from build123d import *

# Parameters (mm, degrees)
BOSS_EXTRUDE1_DEPTH = 3.175


with BuildPart() as part:
    # Sketch1 → Boss-Extrude1 (new body)
    with BuildSketch(Plane.XY):
        with BuildLine():
            Line((-9.525, 12.7), (9.525, 12.7))
            Line((9.525, 12.7), (9.525, 6.35))
            Line((9.525, 6.35), (12.7, 6.35))
            Line((12.7, 6.35), (12.7, 0.865465632))
            ThreePointArc((12.7, 0.865465632), (9.4234, 0), (12.7, -0.865465632))
            Line((12.7, -0.865465632), (12.7, -6.35))
            Line((12.7, -6.35), (9.525, -6.35))
            Line((9.525, -6.35), (9.525, -12.7))
            Line((9.525, -12.7), (6.35, -12.7))
            Line((6.35, -12.7), (6.35, -9.467093743))
            Line((6.35, -9.467093743), (3.175, -9.467093743))
            Line((3.175, -9.467093743), (3.175, -12.7))
            Line((3.175, -12.7), (0.865465632, -12.7))
            ThreePointArc((0.865465632, -12.7), (0, -9.4234), (-0.865465632, -12.7))
            Line((-0.865465632, -12.7), (-3.175, -12.7))
            Line((-3.175, -12.7), (-3.175, -9.467093743))
            Line((-3.175, -9.467093743), (-6.35, -9.467093743))
            Line((-6.35, -9.467093743), (-6.35, -12.7))
            Line((-6.35, -12.7), (-9.525, -12.7))
            Line((-9.525, -12.7), (-9.525, -6.35))
            Line((-9.525, -6.35), (-12.7, -6.35))
            Line((-12.7, -6.35), (-12.7, -0.865465632))
            ThreePointArc((-12.7, -0.865465632), (-9.4234, 0), (-12.7, 0.865465632))
            Line((-12.7, 0.865465632), (-12.7, 6.35))
            Line((-12.7, 6.35), (-9.525, 6.35))
            Line((-9.525, 6.35), (-9.525, 12.7))
        make_face()
    extrude(amount=BOSS_EXTRUDE1_DEPTH)


solid = part.part
The model under review builds one solid part; all positions refer to its coordinate system, in mm. A direction names the side the tool comes from. Give positions to 0.01 mm unless a question says otherwise; leave off trailing zeros. Write each loop counter-clockwise with the first axis right and the second up, starting at its lowest first coordinate (ties: lowest second). Pieces come first, ordered by that corner, then holes.
1. Tool access review of faces 5 (the flat face through (0, 0, 0)), 6 (the flat face through (2, -12.7, 2)), 7 (the flat face through (-6.35, -11, 2)), 8 (the flat face through (9.525, -9, 2)), 9 (the flat face through (11, 6.35, 2)): name each direction out of +Z, -Z, +X, -X, +Y, -Y from which nothing blocks a thin tool from reaching the whole face with its end or side.
2. Wall thickness on L1, parallel to X at y = -11.25, z = 2.5 (3 decimals); L2, parallel to X at y = 8, z = 0.55 (3 decimals); L3, parallel to Y at x = 3.25, z = 2.5: over which ranges is each line inside the solid? List them lowest first.
3. Draft analysis for pull direction X (two halves, no side actions). For faces 1 (the flat face through (5, -9.467, 2)), 2 (the cylindrical face through (-9.425, -0.064, 1.565)), 3 (the flat face through (-11, 6.35, 2)), 4 (the flat face through (-9.525, 9, 2)), state which applies: +X half, -X half, draft (parallel to the pull), parting line (faces both ways), or undercut.
4. Add section B-B, the plane x = -11. Write out the cut boundary in (y, z) (3 decimals), plus the area to 3 significant figures.
5. Add section C-C, the plane y = 0. Write out the cut boundary in (x, z) (3 decimals), plus the area to 3 significant figures.
6. Add section A-A, the plane z = 1.4. Write out the cut boundary in (x, y) (3 decimals), plus the area to 3 significant figures.
7. Add section D-D, the plane x = 0. Write out the cut boundary in (y, z) (3 decimals), plus the area to 3 significant figures.
8. For P1, Ø1, axis at x = 11, z = 1, coming from the +Y side; P2, Ø1, axis at x = -5, z = 2, coming from the -Y side; P3, Ø5.5, axis at x = 0, y = -11.176, coming from the -Z side; P4, Ø1, axis at y = -11.5, z = 1.5, coming from the +X side (3 decimals), all flat-tipped, find the tip position at first contact; note any pin that passes through.
Worked answers:
1. face 5: -Z, +X, -X, +Y, -Y
1. face 6: +Z, -Z, +X, -X, -Y
1. face 7: +Z, -Z, -Y
1. face 8: +Z, -Z, +X, -Y
1. face 9: +Z, -Z, +X, +Y
2. L1: x = -9.525 to -6.35, -3.175 to -1.751, 1.751 to 3.175, 6.35 to 9.525
2. L2: x = -9.525 to 9.525
2. L3: y = -9.47 to 12.7
3. face 1: undercut
3. face 2: undercut
3. face 3: draft
3. face 4: -X half
4. outline: (-6.35, 0) - (-1.744, 0) - (-1.744, 3.175) - (-6.35, 3.175) - close; (1.744, 0) - (6.35, 0) - (6.35, 3.175) - (1.744, 3.175) - close
4. area: 29.2 mm2
5. outline: (-9.423, 0) - (9.423, 0) - (9.423, 3.175) - (-9.423, 3.175) - close
5. area: 59.8 mm2
6. outline: (-12.7, -6.35) - (-9.525, -6.35) - (-9.525, -12.7) - (-6.35, -12.7) - (-6.35, -9.467) - (-3.175, -9.467) - (-3.175, -12.7) - (-0.865, -12.7) arc R1.753 cw (long way) to (0.865, -12.7) - (3.175, -12.7) - (3.175, -9.467) - (6.35, -9.467) - (6.35, -12.7) - (9.525, -12.7) - (9.525, -6.35) - (12.7, -6.35) - (12.7, -0.865) arc R1.753 cw (long way) to (12.7, 0.865) - (12.7, 6.35) - (9.525, 6.35) - (9.525, 12.7) - (-9.525, 12.7) - (-9.525, 6.35) - (-12.7, 6.35) - (-12.7, 0.865) arc R1.753 cw (long way) to (-12.7, -0.865) - close
6. area: 516 mm2
7. outline: (-9.423, 0) - (12.7, 0) - (12.7, 3.175) - (-9.423, 3.175) - close
7. area: 70.2 mm2
8. P1: stops at y = 6.35
8. P2: stops at y = -9.47
8. P3: stops at z = 0
8. P4: stops at x = 9.525
